Can you work these out from the model? Positions are in its coordinate system, mm. Give positions to 0.01 mm unless a question says otherwise; leave off trailing zeros. Loops run counter-clockwise (first coordinate to the right, second up) from the corner with the lowest first, then second, coordinate; pieces in that order, holes last. Notation, with made-up numbers: M 1.25,65.5 L 38.25,65.5 A12 ccw 38.25,80.5 Z; hole C 82,46.5 d9. An arc over 180 degrees is marked long. One line per item, written item: value. Start each with the question number.
from build123d import *

# Parameters (mm, degrees)
SKETCH1_W                  = 381
SKETCH1_H                  = 50.8
BOSS_EXTRUDE1_DEPTH        = 6.35
SKETCH2_R                  = 9.525
CUT_EXTRUDE1_DEPTH         = 193.290749908
F_7_0_201_DIAMETER_HOLE1_D = 5.1054
CIRPATTERN1_COUNT          = 4


with BuildPart() as part:
    # Sketch1 → Boss-Extrude1 (new body)
    with BuildSketch(Plane.XY):
        Rectangle(SKETCH1_W, SKETCH1_H)
    extrude(amount=BOSS_EXTRUDE1_DEPTH)

    # Sketch2 → Cut-Extrude1 (cut, through all)
    with BuildSketch(Plane.XY.offset(6.35)):
        Circle(SKETCH2_R)
    extrude(amount=-CUT_EXTRUDE1_DEPTH, mode=Mode.SUBTRACT)

    # #7 (0.201) Diameter Hole1 (through all)
    with Locations(Plane.XY.offset(6.35)):
        with Locations((17.960512242, 17.960512242)):
            f_7_0_201_diameter_hole1 = Hole(F_7_0_201_DIAMETER_HOLE1_D / 2)

    # CirPattern1: #7 (0.201) Diameter Hole1 ×4 about axis
    cirpattern1_axis = Axis((0, 0, 0), (0, 0, 1))
    for i in range(1, CIRPATTERN1_COUNT):
        add(f_7_0_201_diameter_hole1.rotate(cirpattern1_axis, i * 360 / CIRPATTERN1_COUNT), mode=Mode.SUBTRACT)


solid = part.part
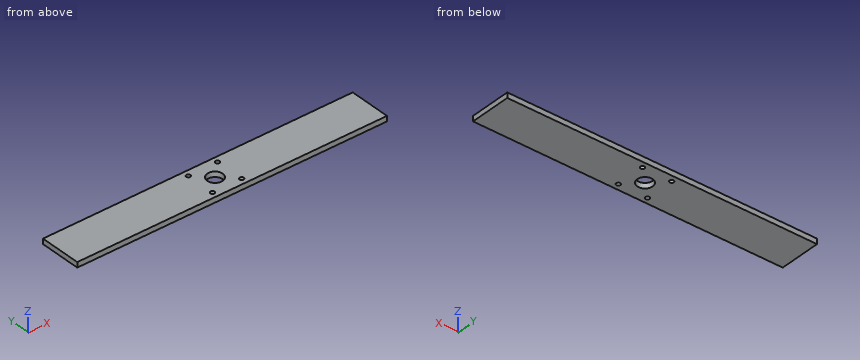
Q1. If we section it at A-A, the plane x = 0: Write out the boundary of the cut face in (y, z) (3 decimals).
Q2. For P1, Ø1, axis at x = 79.5, y = 2.5, coming from the -Z side; P2, Ø3, axis at x = 17.96, y = -17.96, coming from the +Z side, each with a flat end and sliding along its axis, tell me the tip position at first contact or that it passes through.
Q3. I need wall thicknesses on line 1 along X through (y, z) = (-17, 3); line 2 along X through (y, z) = (7, 4.5); line 3 along X through (y, z) = (-3.5, 1.25). Which ranges of each line are inside material? Lowest first, please.
Q4. If we section it at C-C, the plane z = 1.25: Write out the boundary of the cut face in (x, y) (3 decimals), plus the area to 3 significant figures.
Q5. If we section it at B-B, the plane y = 0: Write out the boundary of the cut face in (x, z) (3 decimals).
Response:
1. outline: M -25.4,0 L -9.525,0 L -9.525,6.35 L -25.4,6.35 Z; M 9.525,0 L 25.4,0 L 25.4,6.35 L 9.525,6.35 Z
2. P1: z = 0
2. P2: through
3. line 1: -190.5 to -20.33, -15.6 to 15.6, 20.33 to 190.5
3. line 2: -190.5 to -6.46, 6.46 to 190.5
3. line 3: -190.5 to -8.86, 8.86 to 190.5
4. outline: M -190.5,-25.4 L 190.5,-25.4 L 190.5,25.4 L -190.5,25.4 Z; hole C -17.961,-17.961 d5.105; hole C -17.961,17.961 d5.105; hole C 0,0 d19.05; hole C 17.961,-17.961 d5.105; hole C 17.961,17.961 d5.105
4. area: 19,000 mm^2
5. outline: M -190.5,0 L -9.525,0 L -9.525,6.35 L -190.5,6.35 Z; M 9.525,0 L 190.5,0 L 190.5,6.35 L 9.525,6.35 Z
